Read the model definition and answer for the solid it produces. Units are mm, in the model's axes. Face numbers are marked on the shaded views. A direction names the side the tool comes from. Give positions to 0.01 mm unless a question says otherwise; leave off trailing zeros. Write each loop counter-clockwise with the first axis right and the second up, starting at its lowest first coordinate (ties: lowest second). Pieces come first, ordered by that corner, then holes. Notation, with made-up numbers: (44.25, 25.25) - (92.25, 25.25) arc R25 cw to (92.25, 60.25) - close; hole circle Ø11 at (-8, -36.75). An arc over 180 degrees is marked (long way). Answer as a JSON object with one key per item and string values. Group by question number.
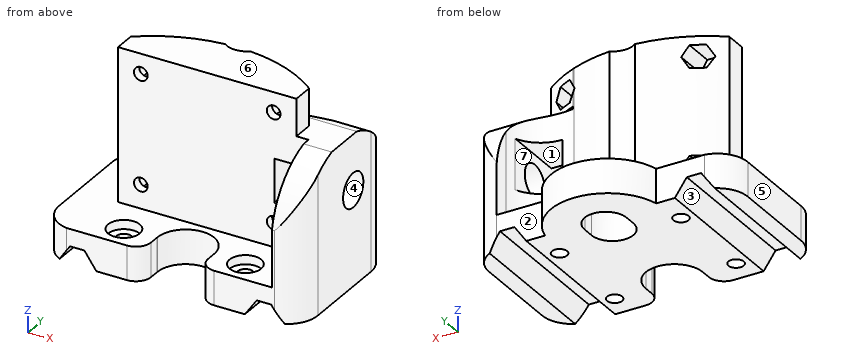
```python
from build123d import *

# Parameters (mm, degrees)
SKETCH1_R                = 2.000043321
SKETCH1_R_2              = 2.000014119
BOSS_EXTRUDE1_DEPTH      = 4.5
CUT_EXTRUDE2_DEPTH       = 46.343813751
SKETCH6_W                = 23.5
SKETCH6_H                = 5.65
BOSS_EXTRUDE2_DEPTH      = 40.25
SKETCH3_R                = 4.181725
CUT_EXTRUDE3_DEPTH       = 2.4
BOSS_EXTRUDE3_DEPTH      = 30.5
SKETCH21_W               = 12.385700762
SKETCH21_H               = 18.597289034
CUT_EXTRUDE16_DEPTH      = 60.959352444
CUT_EXTRUDE20_DEPTH      = 19.55588
CUT_EXTRUDE21_DEPTH      = 64.068406998
CUT_EXTRUDE21_DEPTH_BACK = 64.068406998
SKETCH9_7_R              = 1.8
CUT_EXTRUDE6_DEPTH       = 64.068406998
CUT_EXTRUDE6_DEPTH_BACK  = 4.1004
SKETCH9_R                = 1.8
CUT_EXTRUDE5_DEPTH       = 64.068406927
CUT_EXTRUDE5_DEPTH_BACK  = 64.068406927
SKETCH32_R               = 4.496907104
CUT_EXTRUDE28_DEPTH      = 7.399999239


with BuildPart() as part:
    # Sketch1 → Boss-Extrude1 (new, symmetric)
    with BuildSketch(Plane.XY):
        with BuildLine():
            ThreePointArc((27.3591, -22.750023286), (32.18573506, -20.04264062), (34.100000001, -14.850154064))
            Line((34.100000001, -14.850154064), (34.100000001, 8.850156137))
            ThreePointArc((34.100000001, 8.850156137), (32.18573506, 14.042642693), (27.3591, 16.750025358))
            Line((27.3591, 16.750025358), (14.6356, 16.750025358))
            ThreePointArc((14.6356, 16.750025358), (0, 28.500025358), (-14.6356, 16.750025358))
            Line((-14.6356, 16.750025358), (-27.3591, 16.750025358))
            ThreePointArc((-27.3591, 16.750025358), (-32.18573506, 14.042642693), (-34.100000001, 8.850156137))
            Line((-34.100000001, 8.850156137), (-34.100000001, -14.850154064))
            ThreePointArc((-34.100000001, -14.850154064), (-32.18573506, -20.04264062), (-27.3591, -22.750023286))
            Line((-27.3591, -22.750023286), (-11.500037792, -22.750023286))
            ThreePointArc((-11.500037792, -22.750023286), (-8.671570628, -21.578433826), (-7.499981167, -18.749966661))
            Line((-7.499981167, -18.749966661), (-7.499981167, -16.089239323))
            ThreePointArc((-7.499981167, -16.089239323), (-7.500113179, -16.044739987), (-7.499981167, -16.000240651))
            ThreePointArc((-7.499981167, -16.000240651), (0, -8.544626807), (7.499981167, -16.000240651))
            ThreePointArc((7.499981167, -16.000240651), (7.500113179, -16.044739987), (7.499981167, -16.089239323))
            Line((7.499981167, -16.089239323), (7.499981167, -18.749966661))
            ThreePointArc((7.499981167, -18.749966661), (8.671570628, -21.578433826), (11.500037792, -22.750023286))
            Line((11.500037792, -22.750023286), (27.3591, -22.750023286))
        make_face()
        with Locations((-16.000068831, -16.5)):
            Circle(SKETCH1_R, mode=Mode.SUBTRACT)
        with Locations((16.000068831, -16.5)):
            Circle(SKETCH1_R, mode=Mode.SUBTRACT)
        with Locations((-16.000068831, 7.999981023)):
            Circle(SKETCH1_R_2, mode=Mode.SUBTRACT)
        with Locations((16.000068831, 7.999981023)):
            Circle(SKETCH1_R_2, mode=Mode.SUBTRACT)
    extrude(amount=BOSS_EXTRUDE1_DEPTH, both=True)

    # Sketch4 → Cut-Extrude2 (cut, through all)
    with BuildSketch(Plane.XY.offset(4.5)):
        with BuildLine():
            Line((5.5, 11.5), (5.5, 14.5))
            ThreePointArc((5.5, 14.5), (0, 20), (-5.5, 14.5))
            Line((-5.5, 14.5), (-5.5, 11.5))
            ThreePointArc((-5.5, 11.5), (0, 6), (5.5, 11.5))
        make_face()
    extrude(amount=-CUT_EXTRUDE2_DEPTH, mode=Mode.SUBTRACT)

    # Sketch6 → Boss-Extrude2 (add)
    with BuildSketch(Plane.XY.offset(4.5)):
        with Locations((11.75, -3.625)):
            Rectangle(SKETCH6_W, SKETCH6_H)
        with Locations((-11.75, -3.625)):
            Rectangle(SKETCH6_W, SKETCH6_H)
        with BuildLine():
            Line((0, -0.8), (23.5, -0.8))
            ThreePointArc((23.5, -0.8), (13.984131025, 4.616883926), (3.324005419, 7.118106805))
            ThreePointArc((3.324005419, 7.118106805), (0, 6), (-3.324005419, 7.118106805))
            ThreePointArc((-3.324005419, 7.118106805), (-13.984131025, 4.616883926), (-23.5, -0.8))
            Line((-23.5, -0.8), (0, -0.8))
        make_face()
    extrude(amount=BOSS_EXTRUDE2_DEPTH)

    # Sketch3 → Cut-Extrude3 (cut)
    with BuildSketch(Plane.XY.offset(4.5)):
        with Locations((-16.000068831, 7.999981023)):
            Circle(SKETCH3_R)
        with Locations((16.000068831, 7.999981023)):
            Circle(SKETCH3_R)
        with Locations((16.000068831, -16.500018977)):
            Circle(SKETCH3_R)
        with Locations((-16.000068831, -16.500018977)):
            Circle(SKETCH3_R)
    extrude(amount=-CUT_EXTRUDE3_DEPTH, mode=Mode.SUBTRACT)

    # Sketch15 → Boss-Extrude3 (add)
    with BuildSketch(Plane.XY.offset(4.5)):
        with BuildLine():
            Line((14.314300001, 16.750025358), (14.314300001, -22.750023286))
            Line((14.314300001, -22.750023286), (27.3591, -22.750023286))
            ThreePointArc((27.3591, -22.750023286), (32.18573506, -20.04264062), (34.100000001, -14.850154064))
            Line((34.100000001, -14.850154064), (34.100000001, 8.850156137))
            ThreePointArc((34.100000001, 8.850156137), (32.18573506, 14.042642693), (27.3591, 16.750025358))
            Line((27.3591, 16.750025358), (14.314300001, 16.750025358))
        make_face()
    extrude(amount=BOSS_EXTRUDE3_DEPTH)

    # Sketch21 → Cut-Extrude16 (cut, through all)
    with BuildSketch(Plane.XY.offset(4.5)):
        with Locations((20.507150382, -15.748644517)):
            Rectangle(SKETCH21_W, SKETCH21_H)
        with BuildLine():
            ThreePointArc((27.3591, 12.579600334), (22.93090056, 5.157449584), (14.314300001, 4.485536757))
            Line((14.314300001, 4.485536757), (14.314300001, 16.750025358))
            Line((14.314300001, 16.750025358), (27.3591, 16.750025358))
            Line((27.3591, 16.750025358), (27.3591, 12.579600334))
        make_face()
    extrude(amount=CUT_EXTRUDE16_DEPTH, mode=Mode.SUBTRACT)

    # Sketch22 → Cut-Extrude20 (cut)
    with BuildSketch(Plane(origin=(34.100000001, 0, 0), x_dir=(0, 0, -1), z_dir=(1, 0, 0))):
        with BuildLine():
            Line((-35, 18.44611001), (-35, 2.44611001))
            ThreePointArc((-35, 2.44611001), (-28.722119173, 12.152830277), (-18.115600586, 16.75))
            Line((-18.115600586, 16.75), (-18.115600586, 18.44611001))
            Line((-18.115600586, 18.44611001), (-35, 18.44611001))
        make_face()
        with BuildLine():
            ThreePointArc((-19.450399399, -22.75), (-29.235735953, -17.914679764), (-35, -8.646109581))
            Line((-35, -8.646109581), (-35, -24.646109581))
            Line((-35, -24.646109581), (-19.450399399, -24.646109581))
            Line((-19.450399399, -24.646109581), (-19.450399399, -22.75))
        make_face()
    extrude(amount=-CUT_EXTRUDE20_DEPTH, mode=Mode.SUBTRACT)

    # Sketch24 → Cut-Extrude21 (cut, two sides)
    with BuildSketch(Plane(origin=(0, 0, 0), x_dir=(1, 0, 0), z_dir=(0, 1, 0))) as cut_extrude21_sk:
        Polygon((17.75, -16.135499954), (19.635499954, -14.25), (26.700000763, -14.25), (26.700000763, -27.549999237), (17.75, -27.549999237), align=None)
    extrude(amount=CUT_EXTRUDE21_DEPTH, mode=Mode.SUBTRACT)
    extrude(cut_extrude21_sk.sketch, amount=-CUT_EXTRUDE21_DEPTH_BACK, mode=Mode.SUBTRACT)

    # Sketch9<7> → Cut-Extrude6 (cut, two sides)
    with BuildSketch(Plane(origin=(0, 0, 0), x_dir=(1, 0, 0), z_dir=(0, 1, 0))) as cut_extrude6_sk:
        Polygon((-14.035898385, -39.5), (-15.767949192, -36.5), (-19.232050808, -36.5), (-20.964101615, -39.5), (-19.232050808, -42.5), (-15.767949192, -42.5), align=None)
        with Locations(Location((-17.5, -39.5, 0), (0, 0, 90))):
            Circle(SKETCH9_7_R, mode=Mode.SUBTRACT)
        Polygon((15.767949192, -36.5), (19.232050808, -36.5), (20.964101615, -39.5), (19.232050808, -42.5), (15.767949192, -42.5), (14.035898385, -39.5), align=None)
        with Locations(Location((17.5, -39.5, 0), (0, 0, 90))):
            Circle(SKETCH9_7_R, mode=Mode.SUBTRACT)
        Polygon((14.035898385, -10.744445), (15.767949192, -13.744445), (19.232050808, -13.744445), (20.964101615, -10.744445), (19.232050808, -7.744445), (15.767949192, -7.744445), align=None)
        with Locations(Location((17.5, -10.744445, 0), (0, 0, 90))):
            Circle(SKETCH9_7_R, mode=Mode.SUBTRACT)
        Polygon((-15.767949192, -13.744445), (-19.232050808, -13.744445), (-20.964101615, -10.744445), (-19.232050808, -7.744445), (-15.767949192, -7.744445), (-14.035898385, -10.744445), align=None)
        with Locations(Location((-17.5, -10.744445, 0), (0, 0, 90))):
            Circle(SKETCH9_7_R, mode=Mode.SUBTRACT)
    extrude(amount=CUT_EXTRUDE6_DEPTH, mode=Mode.SUBTRACT)
    extrude(cut_extrude6_sk.sketch, amount=-CUT_EXTRUDE6_DEPTH_BACK, mode=Mode.SUBTRACT)

    # Sketch9 → Cut-Extrude5 (cut, two sides)
    with BuildSketch(Plane(origin=(0, 0, 0), x_dir=(1, 0, 0), z_dir=(0, 1, 0))) as cut_extrude5_sk:
        with Locations(Location((-17.5, -39.5, 0), (0, 0, 90))):
            Circle(SKETCH9_R)
        with Locations(Location((17.5, -39.5, 0), (0, 0, 90))):
            Circle(SKETCH9_R)
        with Locations(Location((-17.5, -10.744445, 0), (0, 0, 90))):
            Circle(SKETCH9_R)
        Polygon((-22.70606608, 0), (-19.555132158, 4.5), (-29.647000001, 4.5), (-26.49606608, 0), align=None)
        Polygon((19.555132158, 4.5), (29.647000001, 4.5), (26.49606608, 0), (22.70606608, 0), align=None)
        with Locations(Location((17.5, -10.744445, 0), (0, 0, 90))):
            Circle(SKETCH9_R)
    extrude(amount=CUT_EXTRUDE5_DEPTH, mode=Mode.SUBTRACT)
    extrude(cut_extrude5_sk.sketch, amount=-CUT_EXTRUDE5_DEPTH_BACK, mode=Mode.SUBTRACT)

    # Sketch32 → Cut-Extrude28 (cut)
    with BuildSketch(Plane(origin=(34.100000001, 0, 0), x_dir=(0, 0, -1), z_dir=(1, 0, 0))):
        with Locations((-20.505386522, 0.902118416)):
            Circle(SKETCH32_R)
    extrude(amount=-CUT_EXTRUDE28_DEPTH, mode=Mode.SUBTRACT)


solid = part.part
```
1) Flat-ended cylindrical pins translate along their axes: pin 1 Ø4 at (x, z) = (17.5, 39.5) entering from +Y; pin 2 Ø1.5 at (y, z) = (13.5, 0.5) entering from -X (3 decimals); pin 3 Ø12 at (x, z) = (3, 31) entering from -Y; pin 4 Ø1 at (x, y) = (-13.5, 21.5) entering from -Z. Find the tip coordinate at first contact, or state that the pin passes through.
2) Find the intervals of material crossed by line 1 (Z direction, x = -17, y = -4); line 2 (X direction, y = -6, z = 39.5); line 3 (Z direction, x = 20, y = -1.5), in increasing order. Write a range as [from, to].
3) Find section C-C, the plane x = -24.5. Write down the section's boundary in (y, z).
4) For a pull along X with two mould halves and no side action, classify the marked faces 5, 6 and 7 as released by +X, released by -X, zero draft, split by the parting line, or undercut.
5) Which of the six approach directions +Z, -Z, +X, -X, +Y, -Y give full straight-line access (tool end or side, diameter ignored) to the marked faces 1, 2, 3 and 4?
6) Find section D-D, the plane z = 30. Write down the section's boundary in (x, y), and give its area (3 significant figures).
7) Find section B-B, the plane x = 28.5. Write down the section's boundary in (y, z), and give its area (3 significant figures).
8) Find section A-A, the plane x = 0. Write down the section's boundary in (y, z).
Values follow:
{
 "1": {"pin 1": "stops at y = -4.1", "pin 2": "stops at x = -33.085", "pin 3": "stops at y = -6.45", "pin 4": "passes through"},
 "2": {"line 1": "z = [-4.5, 7.74], [13.74, 36.5], [42.5, 44.75]", "line 2": "x = [-23.5, -19.3], [-15.7, 15.7], [19.3, 23.5]", "line 3": "z = [-3.86, 9.07], [12.41, 14.25], [27.55, 37.83], [41.17, 44.75]"},
 "3": {"outline": "(-22.75, 0) - (16.75, 0) - (16.75, 4.5) - (-22.75, 4.5) - close"},
 "4": {"face 5": "released by -X", "face 6": "zero draft", "face 7": "undercut"},
 "5": {"face 1": "+Y, -Y", "face 2": "+Z, -Z, +X, +Y", "face 3": "-Z, +Y, -Y", "face 4": "+X"},
 "6": {"outline": "(-23.5, -6.45) - (26.7, -6.45) - (26.7, -17.18) - (33.75, -17.18) arc R8 ccw to (34.1, -14.85) - (34.1, 8.85) arc R8 ccw to (33.81, 10.97) - (27.12, 10.97) arc R9.4 cw to (14.31, 4.49) arc R38.28 ccw to (3.32, 7.12) arc R5.5 cw to (-3.32, 7.12) arc R38.28 ccw to (-23.5, -0.8) - close", "area": "788 mm2"},
 "7": {"outline": "(-22.48, -2.86) - (16.48, -2.86) - (16.48, 19.8) arc R19.96 ccw to (2.45, 35) - (-8.65, 35) arc R19.9 ccw to (-22.48, 20.69) - close; hole circle Ø8.99 at (0.9, 20.51)", "area": "1,280 mm2"},
 "8": {"outline": "(-8.54, -4.5) - (6, -4.5) - (6, 44.75) - (-6.45, 44.75) - (-6.45, 4.5) - (-8.54, 4.5) - close; (20, -4.5) - (28.5, -4.5) - (28.5, 4.5) - (20, 4.5) - close"}
}
